from build123d import *


with BuildPart() as part:
    # Sketch1 → Revolve1 (revolve)
    with BuildSketch(Plane(origin=(0, 0, 0), x_dir=(-1, 0, 0), z_dir=(0, 0, -1)), mode=Mode.PRIVATE) as revolve1_sk:
        with BuildLine():
            Line((-3.997568228, 0.098596016), (-3.826794919, 0))
            Line((-3.826794919, 0), (5.826794919, 0))
            Line((5.826794919, 0), (6, 0.1))
            Line((6, 0.1), (6, 1))
            Line((6, 1), (5.5, 1.5))
            Line((5.5, 1.5), (1, 1.5))
            ThreePointArc((1, 1.5), (0.926794919, 1.426794919), (0.826794919, 1.4))
            Line((0.826794919, 1.4), (0.2, 1.4))
            ThreePointArc((0.2, 1.4), (0.058578644, 1.458578644), (0, 1.6))
            Line((0, 1.6), (0, 2))
            Line((0, 2), (-2, 2))
            ThreePointArc((-2, 2), (-3.37891406, 1.448653173), (-3.997568228, 0.098596016))
        make_face()
    revolve(revolve1_sk.sketch.rotate(Axis((4.002354589, 0, 0), (-1, 0, 0)), 270), axis=Axis((4.002354589, 0, 0), (-1, 0, 0)))


solid = part.part
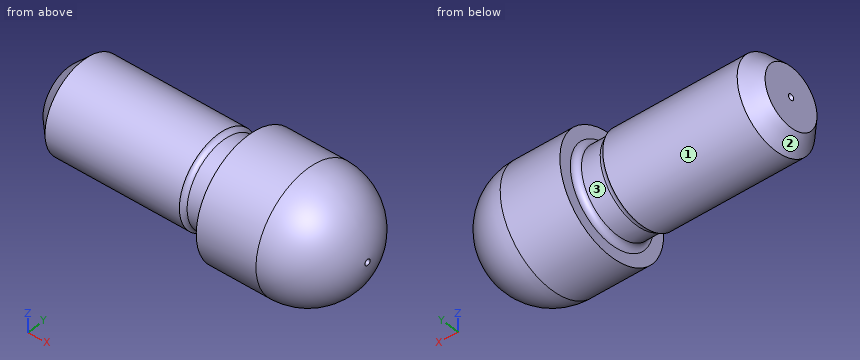
Design review of the part built by this model. Coordinates are the model's own, in mm. Face numbers are marked on the shaded views. Round coordinates to 2 decimals unless told otherwise and drop trailing zeros. Write each loop counter-clockwise with the first axis right and the second up, starting at its lowest first coordinate (ties: lowest second). Pieces come first, ordered by that corner, then holes. Notation, with made-up numbers: (-32.75, 21) -> (4.25, 21) arc R15 cw to (4.25, 42) -> close; hole circle Ø11 at (-30.5, 49). An arc over 180 degrees is marked (long way). One line per question, with ' | ' between items.
(1) Take a section at C-C, the plane x = 1.75. State the section outline as (y, z) points.
Result sheet:
outline: circle Ø4 at (0, 0)
(2) Take a section at A-A, the plane x = -4. State the section outline as (y, z) points.
Result sheet:
outline: circle Ø3 at (0, 0)
(3) Insertion check: P1, Ø1, axis at x = -1.5, y = -1, coming from the -Z side. The pin has a flat end and moves straight along its axis. Give the tip position at first contact, or say it passes through.
Result sheet:
P1: z = -1.41
(4) Wall thickness on line 1 (Z direction, x = -5, y = -0.05); line 2 (Y direction, x = 1.5, z = -0.1); line 3 (Y direction, x = 1.5, z = -1.2): over which ranges is each line inside the solid? List them lowest first. Write a range as [from, to].
Result sheet:
line 1: [-1.5, 1.5] | line 2: [-2, 2] | line 3: [-1.6, 1.6]
(5) Take a section at B-B, the plane y = 1.7. State the section outline as (x, z) points, and give its area (3 significant figures).
Result sheet:
outline: (0, -1.05) -> (2, -1.05) arc R1.05 ccw to (2, 1.05) -> (0, 1.05) -> close | area: 5.96 mm2
(6) Draft analysis for pull direction X (two halves, no side actions). For the marked faces 1, 2 and 3, state which applies: released by +X, released by -X, zero draft, split by the parting line, or undercut.
Result sheet:
face 1: zero draft | face 2: released by -X | face 3: undercut
